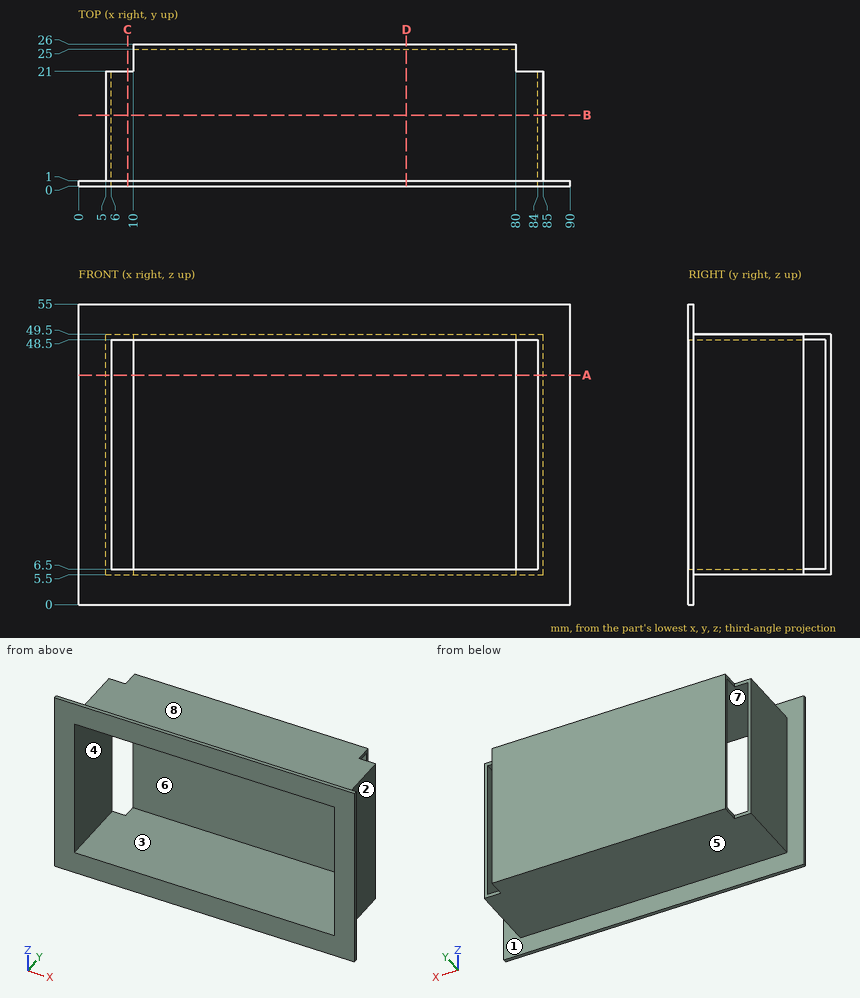
Can you work these out from the drawing? Everything is in mm from the part's minimum corner. A direction names the side the tool comes from. Round coordinates to 2 decimals unless told otherwise and drop trailing zeros. Write each loop counter-clockwise with the first axis right and the second up, starting at its lowest first coordinate (ties: lowest second). Pieces come first, ordered by that corner, then holes.
1. For the marked faces 5, 6, 7 and 8, which set-ups out of +Z, -Z, +X, -X, +Y, -Y let a thin tool reach every point of the face, with its end or its side?
2. I need wall thicknesses on L1, parallel to X at y = 8.5, z = 30.5; L2, parallel to Z at x = 40, y = 2.5; L3, parallel to Y at x = 45.5, z = 18. Which ranges of each line are inside material? Lowest first, please.
3. Suppose I cut it at C-C (x = 9). List the corners of the cut face in (y, z) for me.
4. If we mould it in two halves opening along X, with no side actions, what happens to the marked faces 1, 2, 3 and 4? For each: released by +X, released by -X, zero draft, split by the parting line, or undercut.
5. Suppose I cut it at B-B (y = 13). List the corners of the cut face in (x, z) for me.
6. Suppose I cut it at D-D (x = 60). List the corners of the cut face in (y, z) for me.
7. Suppose I cut it at A-A (z = 42). List the corners of the cut face in (x, y) for me, and give its area (3 significant figures).
8. Will these pins go through, and if not, where does the flat tip stop? pin 1 Ø10 at (y, z) = (12.5, 33.5) entering from -X; pin 2 Ø4 at (y, z) = (23.5, 29.5) entering from -X; pin 3 Ø10 at (x, y) = (29.5, 22) entering from +Z.
Answer sheet:
1. face 5: -Z, +X, -X, +Y
1. face 6: +X, -X, -Y
1. face 7: -Y
1. face 8: +Z, +X, -X, +Y
2. L1: x = 5 to 6, 84 to 85
2. L2: z = 5.5 to 6.5, 48.5 to 49.5
2. L3: y = 25 to 26
3. outline: (0, 0) - (1, 0) - (1, 5.5) - (21, 5.5) - (21, 6.5) - (0, 6.5) - close; (0, 48.5) - (21, 48.5) - (21, 49.5) - (1, 49.5) - (1, 55) - (0, 55) - close
4. face 1: zero draft
4. face 2: released by +X
4. face 3: undercut
4. face 4: undercut
5. outline: (5, 5.5) - (85, 5.5) - (85, 49.5) - (5, 49.5) - close; hole (6, 6.5) - (84, 6.5) - (84, 48.5) - (6, 48.5) - close
6. outline: (0, 0) - (1, 0) - (1, 5.5) - (26, 5.5) - (26, 49.5) - (1, 49.5) - (1, 55) - (0, 55) - (0, 48.5) - (25, 48.5) - (25, 6.5) - (0, 6.5) - close
7. outline: (0, 0) - (6, 0) - (6, 21) - (5, 21) - (5, 1) - (0, 1) - close; (10, 25) - (80, 25) - (80, 26) - (10, 26) - close; (84, 0) - (90, 0) - (90, 1) - (85, 1) - (85, 21) - (84, 21) - close
7. area: 122 mm2
8. pin 1: stops at x = 5
8. pin 2: stops at x = 10
8. pin 3: stops at z = 49.5
